Could you check a few things on this model? Use its own coordinates, in mm. A direction names the side the tool comes from. Round coordinates to 2 decimals unless told otherwise and drop trailing zeros. Write each loop counter-clockwise with the first axis right and the second up, starting at its lowest first coordinate (ties: lowest second). Pieces come first, ordered by that corner, then holes. Notation, with made-up numbers: (52.25, -35.75) -> (74.25, -35.75) arc R20 ccw to (74.25, -6.75) -> close; hole circle Ø6 at (42, 27.5). An arc over 180 degrees is marked (long way). Answer in a Markdown table with one row per item. Add a question column.
Autodesk Inventor part; units mm, degrees
ref_plane "YZ Plane" through (0, 0, 0) normal (1, 0, 0) x (0, 1, 0)
ref_plane "XZ Plane" through (0, 0, 0) normal (0, 1, 0) x (-1, 0, 0)
ref_plane "XY Plane" through (0, 0, 0) normal (0, 0, 1) x (1, 0, 0)
sketch "Sketch1" plane through (0, 0, 0) normal (0, 1, 0) x (-1, 0, 0)
  circle A0 centre (0, 0) radius 15
  circle A1 centre (0, 0) radius 16
  circle A2 centre (0, 0) radius 5.25
  dimension "d0" = 30
  dimension "d1" = 1
  dimension "d6" = 10.5
extrude "Extrusion1" add sketch "Sketch1" along normal blind 20 contours A1
extrude "Extrusion2" add sketch "Sketch1" against normal blind 2 contours A0 | A1
sketch "Sketch3" plane through (0, -2, 0) normal (0, -1, 0) x (1, 0, 0)
  circle A0 centre (0, 0) radius 16
  line L0 (15.1987, 5) -> (40.1987, 5)
  arc A1 (40.1987, -5) -> (40.1987, 5) centre (40.1987, 0) ccw
  line L1 (40.1987, -5) -> (15.1987, -5)
  circle A2 centre (40.1987, 0) radius 2.5
  dimension "d9" = 5
  dimension "d10" = 25
  dimension "d13" = 5
extrude "Extrusion3" add sketch "Sketch3" against normal blind 2 contours A0 L0 A1 L1
properties part number "Pok Mk 3 Yaw Motor Mount"
(1) Suppose I cut it at C-C, the plane z = 4. Please give me the cut outline in (x, y), then the cut area to 3 significant figures.
(2) If we mould it in two halves opening along X, with no side actions, what happens to faces 5 (the face through (45.197, -1.014, -0.11)), 6 (the face through (0, 0, -6)), 7 (the face through (7, -2, 0))? For each: pulls with the +X half, pulls with the -X half, needs draft (parallel to the pull), parting line crosses it, or undercut.
(3) Suppose I cut it at A-A, the plane x = 0. Please give me the cut outline in (y, z).
(4) Suppose I cut it at B-B, the plane z = 0. Please give me the cut outline in (x, y), then the cut area to 3 significant figures.
(5) I need wall thicknesses on L1, parallel to Z at x = 0, y = 15.5; L2, parallel to Y at x = 4.5, z = 3.5; L3, parallel to X at y = 16.75, z = -5.5. Which ranges of each line are inside material? Lowest first, please.
(6) Suppose I cut it at D-D, the plane y = 7.75. Please give me the cut outline in (x, z).
(7) On a 3-axis mill with a long thin cutter (end or side, diameter ignored), from which of +Z, -Z, +X, -X, +Y, -Y can I reach the whole of each face in a straight line? I mean faces 1 (the face through (14.985, 9.86, -0.66)), 2 (the face through (28, -1, -5)), 3 (the face through (37.7, -1, 0.1)), 4 (the face through (28, -1, 5)). Say none if no direction works.
(8) For P1, Ø4, axis at x = 23.5, z = -4.5, coming from the +Y side; P2, Ø5, axis at y = 17, z = 11.5, coming from the +X side; P3, Ø1, axis at x = 25.5, y = -0.5, coming from the -Z side, each with a flat end and sliding along its axis, tell me the tip position at first contact or that it passes through.
Response:
| question | item | result |
|---|---|---|
| 1 | outline | (-15.49, -2) -> (-3.4, -2) -> (-3.4, 0) -> (-14.46, 0) -> (-14.46, 20) -> (-15.49, 20) -> close; (3.4, -2) -> (43.2, -2) -> (43.2, 0) -> (15.49, 0) -> (15.49, 20) -> (14.46, 20) -> (14.46, 0) -> (3.4, 0) -> close |
| 1 | area | 145 mm² |
| 2 | face 5 | pulls with the +X half |
| 2 | face 6 | undercut |
| 2 | face 7 | needs draft |
| 3 | outline | (-2, -16) -> (20, -16) -> (20, -15) -> (0, -15) -> (0, -5.25) -> (-2, -5.25) -> close; (-2, 5.25) -> (0, 5.25) -> (0, 15) -> (20, 15) -> (20, 16) -> (-2, 16) -> close |
| 4 | outline | (-16, -2) -> (-5.25, -2) -> (-5.25, 0) -> (-15, 0) -> (-15, 20) -> (-16, 20) -> close; (5.25, -2) -> (37.7, -2) -> (37.7, 0) -> (16, 0) -> (16, 20) -> (15, 20) -> (15, 0) -> (5.25, 0) -> close; (42.7, -2) -> (45.2, -2) -> (45.2, 0) -> (42.7, 0) -> close |
| 4 | area | 131 mm² |
| 5 | L1 | -16 to -15, 15 to 16 |
| 5 | L2 | -2 to 0 |
| 5 | L3 | -15.02 to -13.96, 13.96 to 15.02 |
| 6 | outline | circle Ø32 at (0, 0); hole circle Ø30 at (0, 0) |
| 7 | face 1 | +Y |
| 7 | face 2 | -Z, +X, +Y, -Y |
| 7 | face 3 | +Y, -Y |
| 7 | face 4 | +Z, +X, +Y, -Y |
| 8 | P1 | y = 0 |
| 8 | P2 | x = 13.23 |
| 8 | P3 | z = -5 |
